```python
from build123d import *

# Parameters (mm, degrees)
SKETCH2_R           = 14.9
SKETCH2_R_2         = 1.7
BOSS_EXTRUDE1_DEPTH = 50
SKETCH3_R           = 2.1
CUT_EXTRUDE1_DEPTH  = 5.7


with BuildPart() as part:
    # Sketch2 → Boss-Extrude1 (new body)
    with BuildSketch(Plane.XY):
        Circle(SKETCH2_R)
        with Locations((0, 7)):
            Circle(SKETCH2_R_2, mode=Mode.SUBTRACT)
        with Locations((6.062177826, -3.5)):
            Circle(SKETCH2_R_2, mode=Mode.SUBTRACT)
        with Locations((-6.062177826, -3.5)):
            Circle(SKETCH2_R_2, mode=Mode.SUBTRACT)
    extrude(amount=BOSS_EXTRUDE1_DEPTH)

    # Sketch3 → Cut-Extrude1 (cut)
    with BuildSketch(Plane.XY.offset(50)):
        with Locations((0, 7)):
            Circle(SKETCH3_R)
        with Locations((6.062177826, -3.5)):
            Circle(SKETCH3_R)
        with Locations((-6.062177826, -3.5)):
            Circle(SKETCH3_R)
    cut_extrude1 = extrude(amount=-CUT_EXTRUDE1_DEPTH, mode=Mode.SUBTRACT)

    # Mirror1: Cut-Extrude1 across plane
    add(cut_extrude1.mirror(Plane.XY.offset(25)), mode=Mode.SUBTRACT)


solid = part.part
```
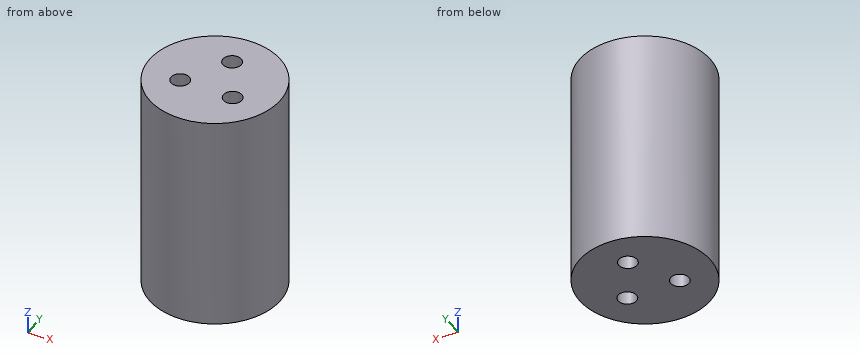
The listing builds one solid part. Answer for the finished solid, in the listing's coordinates (mm). Round coordinates to 2 decimals unless told otherwise and drop trailing zeros. Write each loop counter-clockwise with the first axis right and the second up, starting at its lowest first coordinate (ties: lowest second). Pieces come first, ordered by that corner, then holes. Notation, with made-up numbers: (-7.5, 39.25) -> (5.5, 39.25) arc R35 ccw to (5.5, 78.25) -> close; hole circle Ø11 at (37.25, -4.5). An arc over 180 degrees is marked (long way). Use CSV: the item, a comma, the result in double quotes. Start each with the question number.
(1) Section D-D on z = 37.5 is taken. Give the vertices of the cut face in (x, y), then the cut area to 3 significant figures.
(2) Section A-A on x = 0 is taken. Give the vertices of the cut face in (y, z), then the cut area to 3 significant figures.
(3) Each of these flat-tipped pins is pushed along its axis until it touches: pin 1 (3.5 mm diameter, centred on x = 6, y = -3.5, fed in from -Z); pin 2 (3 mm diameter, centred on x = 3.5, z = 7, fed in from -Y); pin 3 (2 mm diameter, centred on x = 7, y = -4, fed in from +Z); pin 4 (2.5 mm diameter, centred on x = 6.06, y = -3.5, fed in from -Z). Where does it stop, or does it pass through?
(4) Section C-C on y = 6 is taken. Give the vertices of the cut face in (x, z), then the cut area to 3 significant figures.
(5) Consider L1, parallel to Y at x = 0, z = 26; L2, parallel to Y at x = 0, z = 3; L3, parallel to X at y = 7.25, z = 13. Determine where each line is inside the solid, lowest interval first. Write a range as from..to.
(6) Section B-B on y = -3.5 is taken. Give the vertices of the cut face in (x, z), then the cut area to 3 significant figures.
A:
1,outline,"circle Ø29.8 at (0, 0); hole circle Ø3.4 at (-6.06, -3.5); hole circle Ø3.4 at (0, 7); hole circle Ø3.4 at (6.06, -3.5)"
1,area,"670 mm²"
2,outline,"(-14.9, 0) -> (4.9, 0) -> (4.9, 5.7) -> (5.3, 5.7) -> (5.3, 44.3) -> (4.9, 44.3) -> (4.9, 50) -> (-14.9, 50) -> close; (8.7, 5.7) -> (9.1, 5.7) -> (9.1, 0) -> (14.9, 0) -> (14.9, 50) -> (9.1, 50) -> (9.1, 44.3) -> (8.7, 44.3) -> close"
2,area,"1,310 mm²"
3,pin 1,"stops at z = 5.7"
3,pin 2,"stops at y = -14.77"
3,pin 3,"stops at z = 44.3"
3,pin 4,"passes through"
4,outline,"(-13.64, 0) -> (-1.85, 0) -> (-1.85, 5.7) -> (-1.37, 5.7) -> (-1.37, 44.3) -> (-1.85, 44.3) -> (-1.85, 50) -> (-13.64, 50) -> close; (1.37, 5.7) -> (1.85, 5.7) -> (1.85, 0) -> (13.64, 0) -> (13.64, 50) -> (1.85, 50) -> (1.85, 44.3) -> (1.37, 44.3) -> close"
4,area,"1,220 mm²"
5,L1,"y = -14.9..5.3, 8.7..14.9"
5,L2,"y = -14.9..4.9, 9.1..14.9"
5,L3,"x = -13.02..-1.68, 1.68..13.02"
6,outline,"(-14.48, 0) -> (-8.16, 0) -> (-8.16, 5.7) -> (-7.76, 5.7) -> (-7.76, 44.3) -> (-8.16, 44.3) -> (-8.16, 50) -> (-14.48, 50) -> close; (-4.36, 5.7) -> (-3.96, 5.7) -> (-3.96, 0) -> (3.96, 0) -> (3.96, 5.7) -> (4.36, 5.7) -> (4.36, 44.3) -> (3.96, 44.3) -> (3.96, 50) -> (-3.96, 50) -> (-3.96, 44.3) -> (-4.36, 44.3) -> close; (7.76, 5.7) -> (8.16, 5.7) -> (8.16, 0) -> (14.48, 0) -> (14.48, 50) -> (8.16, 50) -> (8.16, 44.3) -> (7.76, 44.3) -> close"
6,area,"1,090 mm²"
